Read the model definition and answer for the solid it produces. Units are mm, in the model's axes. Coordinates: 2 decimals unless noted, no trailing zeros. Order: outer loops, then holes, each group sorted by start corner. A loop starts at its lowest first (then second) coordinate and runs counter-clockwise, first axis right, second up.
```python
from build123d import *

# Parameters (mm, degrees)
CROQUIS1_W                   = 30
CROQUIS1_H                   = 10
SALIENTE_EXTRUIR1_DEPTH      = 2
SALIENTE_EXTRUIR2_DEPTH      = 2
SALIENTE_EXTRUIR2_DEPTH_BACK = 2
CROQUIS2_W                   = 30
CROQUIS2_H                   = 2
CHAFL_N1_SIZE                = 2
REDONDEO1_R                  = 3
CORTAR_EXTRUIR1_DEPTH        = 1.3


with BuildPart() as part:
    # Croquis1 → Saliente-Extruir1 (new body)
    with BuildSketch(Plane(origin=(0, 0, 0), x_dir=(1, 0, 0), z_dir=(0, 1, 0))):
        Rectangle(CROQUIS1_W, CROQUIS1_H)
    extrude(amount=SALIENTE_EXTRUIR1_DEPTH)

    # Croquis2 → Saliente-Extruir2 (add, two sides: drawn at the far end of the back side and taken through both)
    with BuildSketch(Plane(origin=(0, 2, 0), x_dir=(1, 0, 0), z_dir=(0, 1, 0)).offset(-SALIENTE_EXTRUIR2_DEPTH_BACK)):
        with Locations((0, 6)):
            Rectangle(CROQUIS2_W, CROQUIS2_H)
    extrude(amount=SALIENTE_EXTRUIR2_DEPTH + SALIENTE_EXTRUIR2_DEPTH_BACK)

    # Chaflán1
    chafl_n1_edges = [part.edges().sort_by_distance(p)[0] for p in [
        (0, 0, 5),
    ]]
    chamfer(chafl_n1_edges, length=CHAFL_N1_SIZE - 0.0001)  # a hair under: the kernel refuses the full size

    # Redondeo1
    redondeo1_edges = [part.edges().sort_by_distance(p)[0] for p in [
        (0, 0, -7),
    ]]
    fillet(redondeo1_edges, radius=REDONDEO1_R)

    # Croquis3 → Cortar-Extruir1 (cut)
    with BuildSketch(Plane.XZ):
        Polygon((-9.961494987, -0.07018817), (-8.709002423, 1.683238665), (-7.549155707, 1.683238665), (-7.549155707, -3.398633507), (-8.83001578, -3.398633507), (-8.83001578, -0.22414092), (-9.330931139, -0.930250522), align=None)
        Polygon((-11.80023979, 1.683238665), (-13, 1.683238665), (-13, -3.398633507), (-11.724069575, -3.398633507), (-11.724069575, -0.22414092), (-10.233410768, -2.257336324), (-9.583176724, -1.340741346), align=None)
        with BuildLine():
            Line((-6.600409237, 1.683238665), (-6.600409237, -1.725226293))
            ThreePointArc((-6.600409237, -1.725226293), (-4.45912989, -3.411949657), (-2.317850543, -1.725226293))
            Line((-2.317850543, -1.725226293), (-2.317850543, 1.683238665))
            Line((-2.317850543, 1.683238665), (-3.56164133, 1.683238665))
            Line((-3.56164133, 1.683238665), (-3.56164133, -1.725226293))
            ThreePointArc((-3.56164133, -1.725226293), (-4.455396596, -2.280675862), (-5.349151863, -1.725226293))
            Line((-5.349151863, -1.725226293), (-5.349151863, 1.683238665))
            Line((-5.349151863, 1.683238665), (-6.600409237, 1.683238665))
        make_face()
        Polygon((-0.147635828, -1.165769584), (-1.416632441, 0.454814455), (-1.416632441, -3.411949657), (-0.147635828, -3.411949657), align=None)
        Polygon((-1.416632441, 1.126001398), (-1.416632441, 1.683238665), (-0.354158469, 1.683238665), (3.073485226, -2.863879645), (3.073485226, -3.411949657), (2.004100926, -3.411949657), align=None)
        Polygon((1.874218963, -0.552422461), (1.874218963, 1.683238665), (3.073485226, 1.683238665), (3.073485226, -2.083956703), align=None)
        Polygon((6.967028865, 1.683238665), (5.642411569, 1.683238665), (3.668591411, -3.411949657), (4.971319865, -3.411949657), (6.315646772, 0.454814455), (7.616337035, -3.411949657), (8.919127609, -3.411949657), align=None)
        Polygon((9.744634122, -1.460252001), (7.972604821, 1.683238665), (9.46859716, 1.683238665), (10.442731706, -0.22414092), (11.480463321, 1.683238665), (12.951143356, 1.683238665), (11.048523586, -1.460252001), (11.048523586, -3.411949657), (9.744634122, -3.411949657), align=None)
    extrude(amount=-CORTAR_EXTRUIR1_DEPTH, mode=Mode.SUBTRACT)


solid = part.part
```
1) Determine the mould class of faces 1 (the cylindrical face through (0.21, 0.86, -6.1)), 2 (the flat face through (10.954, 0.641, 0.716)) for opening direction Z: pulls with the +Z half, pulls with the -Z half, needs draft (parallel to the pull), parting line crosses it, or undercut.
A:
face 1: pulls with the -Z half
face 2: undercut
2) Straight lines are drawn through the part: line 1 (Z direction, x = 6, y = 3.85); line 2 (Y direction, x = 10, z = 0.25); line 3 (Z direction, x = -0.5, y = 0.8). For each, find the intervals that lie inside material, in ascending order.
A:
line 1: z = -7 to -5
line 2: y = 1.3 to 2
line 3: z = -6.04 to -3.41, -0.72 to -0.09, 1.68 to 3.8
3) A cutting plane is placed at D-D, the plane y = 0.35. State how many separate pieces and enclosed holes the cut face has, and give its area (3 significant figures).
A:
separate pieces: 1
enclosed holes: 8
area: 195 mm2
4) A cutting plane is placed at B-B, the plane y = 3.7. Determine the outline of the cut face in (x, z).
A:
outline: (-15, -7) - (15, -7) - (15, -5) - (-15, -5) - close
5) Flat-ended cylindrical pins translate along their axes: pin 1 Ø2.5 at (x, z) = (10, -1.5) entering from -Y; pin 2 Ø1 at (x, y) = (-6, 0.5) entering from -Z; pin 3 Ø1 at (x, y) = (10.5, 1) entering from +Z; pin 4 Ø1.3 at (x, y) = (2.5, 1) entering from -Z. Find the tip coordinate at first contact, or state that the pin passes through.
A:
pin 1: stops at y = 0
pin 2: stops at z = -6.24
pin 3: stops at z = 4.5
pin 4: stops at z = -6.68
6) A cutting plane is placed at C-C, the plane z = 2.25. Determine the outline of the cut face in (x, y).
A:
outline: (-15, 0) - (15, 0) - (15, 2) - (-15, 2) - close
